Build history of the part. All positions in model axes, mm. A direction names the side the tool comes from. Coordinates: 2 decimals unless noted, no trailing zeros. Order: outer loops, then holes, each group sorted by start corner. A loop starts at its lowest first (then second) coordinate and runs counter-clockwise, first axis right, second up. Notation, with made-up numbers: (27.25, 83) -> (52.25, 83) arc R23 cw to (52.25, 108) -> close; hole circle Ø5 at (40.5, 6). An arc over 180 degrees is marked (long way). Write each question's results on one line, items separated by ' | '.
from build123d import *

# Parameters (mm, degrees)
SKETCH010_W  = 45
SKETCH010_H  = 40
PAD005_DEPTH = 60
SKETCH012_W  = 38.2
SKETCH012_H  = 36.8
SKETCH003_R  = 5.4
SKETCH011_R  = 4.4
SKETCH046_R  = 0.8


with BuildPart() as part:
    # Sketch010 → Pad005 (new body)
    with BuildSketch(Plane.XY):
        with Locations((-40.3, 0)):
            Rectangle(SKETCH010_W, SKETCH010_H)
    extrude(amount=PAD005_DEPTH)

    # SubtractivePipe002: sweep along a path in Sketch028
    with BuildLine(Plane.XZ) as subtractivepipe002_path:
        Line((-39, 9), (-39, 60))
    # Sketch012 → SubtractivePipe002 (sweep, cut)
    with BuildSketch(Plane.XY.offset(9)):
        with Locations((-42.1, 0)):
            Rectangle(SKETCH012_W, SKETCH012_H)
    sweep(path=subtractivepipe002_path.line, mode=Mode.SUBTRACT)

    # Sketch003 (on Face10 of SubtractivePipe) → SubtractiveLoft section 0
    with BuildSketch(Plane(origin=(-17.3, 0, 0), x_dir=(0, -1, 0), z_dir=(-1, 0, 0))):
        with Locations((0, 11)):
            Circle(SKETCH003_R)
    # Sketch011 → SubtractiveLoft section 1
    with BuildSketch(Plane(origin=(-27.8, 0, 0), x_dir=(-0.001529, -0.999998, -0.001524), z_dir=(-0.999994, 0.001524, 0.003058))):
        with Locations((0, 11)):
            Circle(SKETCH011_R)
    loft(mode=Mode.SUBTRACT)

    # SubtractivePipe003: sweep along a path in Sketch034
    with BuildLine(Plane.YZ.offset(-17.8)) as subtractivepipe003_path:
        Line((-20, 4), (20, 4))
    # Sketch033 → SubtractivePipe003 (sweep, cut)
    with BuildSketch(Plane.XZ.offset(20)):
        Polygon((-17.8, 0), (-19.3, 0), (-19.3, 3.5), (-17.8, 5.5), align=None)
    sweep(path=subtractivepipe003_path.line, mode=Mode.SUBTRACT)

    # SubtractivePipe004: sweep along a path in Sketch037
    with BuildLine(Plane.YZ.offset(-17.8)) as subtractivepipe004_path:
        Line((-20, 36), (20, 36))
    # Sketch036 → SubtractivePipe004 (sweep, cut)
    with BuildSketch(Plane.XZ.offset(20)):
        Polygon((-21, 60), (-21, 21), (-17.8, 18), (-17.8, 60), align=None)
    sweep(path=subtractivepipe004_path.line, mode=Mode.SUBTRACT)

    # SubtractivePipe007: sweep along a path in Sketch045
    with BuildLine(Plane.YZ.offset(-17.8)) as subtractivepipe007_path:
        CenterArc((0, 11), 5.4, 0, 360)
    # Sketch046 → SubtractivePipe007 (sweep, cut)
    with BuildSketch(Plane(origin=(0, -2.3, 10.5), x_dir=(1, 0, 0), z_dir=(0, 0, 1))):
        with Locations((-20, -3.12)):
            Circle(SKETCH046_R)
    sweep(path=subtractivepipe007_path.line, mode=Mode.SUBTRACT)


solid = part.part
Item 1: Slice it at A-A, the plane z = 24. List the corners of the cut face in (x, y).
Answer:
outline: (-62.8, -20) -> (-21, -20) -> (-21, 20) -> (-62.8, 20) -> close; hole (-61.2, -18.4) -> (-23, -18.4) -> (-23, 18.4) -> (-61.2, 18.4) -> close
Item 2: Tool access for faces 4 (the flat face through (-41, -20, 30)), 5 (the flat face through (-61.2, 0, 35)), 6 (the flat face through (-21, 0, 41)): list every direction of +Z, -Z, +X, -X, +Y, -Y with a clear straight run to the whole face (end or side of a thin tool).
Answer:
face 4: +Z, -Z, +X, -X, -Y | face 5: +Z | face 6: +Z, +X, +Y, -Y
Item 3: Pin check, flat tips, straight feed: pin 1 (18.5 mm diameter, centred on x = -45.5, y = -5.5, fed in from +Z); pin 2 (4 mm diameter, centred on y = -7.5, z = 42, fed in from +X). Stop position of each tip, or through.
Answer:
pin 1: stops at z = 9 | pin 2: stops at x = -21
Item 4: Drill centre lines: line 1 (X direction, y = 17.5, z = 17); line 2 (X direction, y = 10.5, z = 39); line 3 (Y direction, x = -56, z = 14). Where is each one in solid material? Low to high. Write a range as from..to.
Answer:
line 1: x = -62.8..-61.2, -23..-17.8 | line 2: x = -62.8..-61.2, -23..-21 | line 3: y = -20..-18.4, 18.4..20
Item 5: Slice it at C-C, the plane x = -29. List the corners of the cut face in (y, z), and give its area (3 significant figures).
Answer:
outline: (-20, 0) -> (20, 0) -> (20, 60) -> (18.4, 60) -> (18.4, 9) -> (-18.4, 9) -> (-18.4, 60) -> (-20, 60) -> close | area: 523 mm^2
Item 6: Pull direction X, two halves, no side cores. Call faces 1 (the flat face through (-62.8, 0, 30)), 2 (the flat face through (-23, 0, 35)), 3 (the flat face through (-19.3, 0, 2)): released by +X, released by -X, zero draft, split by the parting line, or undercut.
Answer:
face 1: released by -X | face 2: undercut | face 3: released by +X
Item 7: Slice it at B-B, the plane y = -10. List the corners of the cut face in (x, z), and give its area (3 significant figures).
Answer:
outline: (-62.8, 0) -> (-19.3, 0) -> (-19.3, 3.5) -> (-17.8, 5.5) -> (-17.8, 18) -> (-21, 21) -> (-21, 60) -> (-23, 60) -> (-23, 9) -> (-61.2, 9) -> (-61.2, 60) -> (-62.8, 60) -> close | area: 615 mm^2
